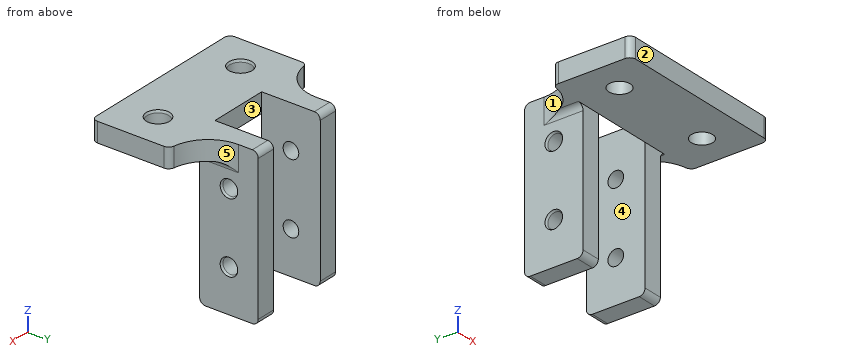
```python
from build123d import *

# Parameters (mm, degrees)
SKETCH1_W                           = 45
SKETCH1_H                           = 20
BOSS_EXTRUDE1_DEPTH                 = 5
BOSS_EXTRUDE2_DEPTH                 = 15
F_4_0_4_DIAMETER_HOLE1_AT_2_COUNT   = 2
F_4_0_4_DIAMETER_HOLE1_AT_2_PITCH   = 18
F_5_5_5_5_DIAMETER_HOLE2_AT_2_COUNT = 2
F_5_5_5_5_DIAMETER_HOLE2_AT_2_PITCH = 27
FILLET1_R                           = 10
FILLET2_R                           = 1.5


with BuildPart() as part:
    # Sketch1 → Boss-Extrude1 (new body)
    with BuildSketch(Plane.XY):
        Rectangle(SKETCH1_W, SKETCH1_H)
    extrude(amount=BOSS_EXTRUDE1_DEPTH)

    # Sketch3 → Boss-Extrude2 (add)
    with BuildSketch(Plane(origin=(0, 10, 0), x_dir=(1, 0, 0), z_dir=(0, 1, 0))):
        Polygon((-7.65, 0), (-7.65, -5), (-12.65, -5), (-12.65, 35), (-7.65, 35), align=None)
        Polygon((7.65, -5), (12.65, -5), (12.65, 35), (7.65, 35), (7.65, 0), align=None)
    extrude(amount=BOSS_EXTRUDE2_DEPTH)

    # Sketch8 → Ø4.0 (4) Diameter Hole1 (revolve, cut)
    with BuildSketch(Plane(origin=(-12.65, 17.5, -24), x_dir=(0, 0, 1), z_dir=(0, 1, 0))):
        Polygon((0, 0), (0, 5), (2, 5), (2, 0.603553391), (2.25, 0), align=None)
    f_4_0_4_diameter_hole1 = revolve(axis=Axis((-19, 17.5, -24), (1, 0, 0)), mode=Mode.SUBTRACT)

    # Ø4.0 (4) Diameter Hole1 at 2: Ø4.0 (4) Diameter Hole1 ×2
    with Locations(*[(0, 0, i * F_4_0_4_DIAMETER_HOLE1_AT_2_PITCH) for i in range(1, F_4_0_4_DIAMETER_HOLE1_AT_2_COUNT)]):
        add(f_4_0_4_diameter_hole1, mode=Mode.SUBTRACT)

    # Mirror3: Ø4.0 (4) Diameter Hole1 across plane
    add(f_4_0_4_diameter_hole1.mirror(Plane(origin=(0, 0, 0), x_dir=(0, 0, 1), z_dir=(1, 0, 0))), mode=Mode.SUBTRACT)

    # Mirror3 copy 1 sketch → Mirror3 copy 1 (revolve, cut)
    with BuildSketch(Plane(origin=(12.65, 17.5, -6), x_dir=(0, 0, 1), z_dir=(0, 1, 0))):
        Polygon((0, 0), (0, -5), (2, -5), (2, -0.603553391), (2.25, 0), align=None)
    revolve(axis=Axis((19, 17.5, -6), (1, 0, 0)), mode=Mode.SUBTRACT)

    # Sketch12 → Ø5.5 (5.5) Diameter Hole2 (revolve, cut)
    with BuildSketch(Plane(origin=(13.5, 0, 5), x_dir=(0, -1, 0), z_dir=(1, 0, 0))):
        Polygon((0, 0), (0, 5), (2.75, 5), (2.75, 0.603553391), (3, 0), align=None)
    f_5_5_5_5_diameter_hole2 = revolve(axis=Axis((13.5, 0, 11.35), (0, 0, -1)), mode=Mode.SUBTRACT)

    # Ø5.5 (5.5) Diameter Hole2 at 2: Ø5.5 (5.5) Diameter Hole2 ×2
    with Locations(*[(-i * F_5_5_5_5_DIAMETER_HOLE2_AT_2_PITCH, 0, 0) for i in range(1, F_5_5_5_5_DIAMETER_HOLE2_AT_2_COUNT)]):
        add(f_5_5_5_5_diameter_hole2, mode=Mode.SUBTRACT)

    # Fillet1
    # the kernel refuses this fillet: 10 mm, written as the material it adds along each edge
    with BuildSketch(Plane(origin=(12.65, 10, 5), x_dir=(1, 0, 0), z_dir=(0, 0, -1))) as fillet1_piece_1:
        with BuildLine():
            CenterArc((10, -9.998874937), FILLET1_R, 90.859468925, 89.140531075)
            Line((0, -9.998874937), (0, 0))
            Line((0, 0), (9.85, 0))
        make_face()
    extrude(amount=5)
    with BuildSketch(Plane(origin=(-12.65, 10, 5), x_dir=(-1, 0, 0), z_dir=(0, 0, -1))) as fillet1_piece_2:
        with BuildLine():
            CenterArc((10, 9.998874937), FILLET1_R, 180, 89.140531075)
            Line((0, 9.998874937), (0, 0))
            Line((0, 0), (9.85, 0))
        make_face()
    extrude(amount=5)

    # Fillet2
    fillet2_edges = [part.edges().sort_by_distance(p)[0] for p in [
        (-10.15, 10, -35),
        (-10.15, 25, -35),
        (-10.15, 25, 5),
        (10.15, 10, -35),
        (10.15, 25, 5),
        (10.15, 25, -35),
        (22.5, -10, 2.5),
        (-22.5, -10, 2.5),
        (-22.5, 10, 2.5),
        (22.5, 10, 2.5),
        (12.65, 14.999437468, 0),
        (-12.65, 14.999437468, 0),
    ]]
    fillet(fillet2_edges, radius=FILLET2_R)


solid = part.part
```
Could you check a few things on this model? Use its own coordinates, in mm. Face numbers are marked on the shaded views. A direction names the side the tool comes from. Round coordinates to 2 decimals unless told otherwise and drop trailing zeros. Loops run counter-clockwise (first coordinate to the right, second up) from the corner with the lowest first, then second, coordinate; pieces in that order, holes last. Notation, with made-up numbers: (12, -26) -> (55, -26) arc R12 cw to (55, -14) -> close; hole circle Ø1 at (76.5, 78). An arc over 180 degrees is marked (long way). One line per question, with ' | ' between items.
(1) For pin 1 Ø1.5 at (y, z) = (13, 0.5) entering from -X; pin 2 Ø2.5 at (y, z) = (17.5, -24) entering from +X; pin 3 Ø7.5 at (y, z) = (19, -18.5) entering from +X; pin 4 Ø3 at (x, z) = (9.5, -11) entering from -Y, each with a flat end and sliding along its axis, tell me the tip position at first contact or that it passes through.
Model answer:
pin 1: stops at x = -16.33 | pin 2: passes through | pin 3: stops at x = 12.65 | pin 4: stops at y = 10
(2) Thinking about a two-plate mould opening in X: for the marked faces 1, 2 and 3, which applies, released by +X, released by -X, zero draft, split by the parting line, or undercut?
Model answer:
face 1: released by -X | face 2: zero draft | face 3: undercut
(3) If we section it at A-A on z = -6: List the corners of the cut face in (x, y) for me.
Model answer:
outline: (-12.65, 10) -> (-7.65, 10) -> (-7.65, 15.5) -> (-12.05, 15.5) -> (-12.65, 15.25) -> close; (-12.65, 19.75) -> (-12.05, 19.5) -> (-7.65, 19.5) -> (-7.65, 25) -> (-12.65, 25) -> close; (7.65, 10) -> (12.65, 10) -> (12.65, 15.25) -> (12.05, 15.5) -> (7.65, 15.5) -> close; (7.65, 19.5) -> (12.05, 19.5) -> (12.65, 19.75) -> (12.65, 25) -> (7.65, 25) -> close
(4) If we section it at D-D on y = 0: List the corners of the cut face in (x, z) for me.
Model answer:
outline: (-22.5, 0) -> (-16.25, 0) -> (-16.25, 4.4) -> (-16.5, 5) -> (-22.5, 5) -> close; (-10.75, 0) -> (10.75, 0) -> (10.75, 4.4) -> (10.5, 5) -> (-10.5, 5) -> (-10.75, 4.4) -> close; (16.25, 0) -> (22.5, 0) -> (22.5, 5) -> (16.5, 5) -> (16.25, 4.4) -> close
(5) If we section it at C-C on z = -14: List the corners of the cut face in (x, y) for me.
Model answer:
outline: (-12.65, 10) -> (-7.65, 10) -> (-7.65, 25) -> (-12.65, 25) -> close; (7.65, 10) -> (12.65, 10) -> (12.65, 25) -> (7.65, 25) -> close
(6) For the marked faces 4 and 5, which set-ups out of +Z, -Z, +X, -X, +Y, -Y let a thin tool reach every point of the face, with its end or its side?
Model answer:
face 4: +Z, -Z, +Y | face 5: +Z, -Z, +X, +Y
(7) If I drill on probe 1 along Z at (x, y) = (10.7, 17.5); probe 2 along X at (y, z) = (0, 2); probe 3 along X at (y, z) = (16.5, -11), over which ranges is the centre line in solid material (lowest first)?
Model answer:
probe 1: z = -35 to -26, -22 to -8, -4 to 5 | probe 2: x = -22.5 to -16.25, -10.75 to 10.75, 16.25 to 22.5 | probe 3: x = -12.65 to -7.65, 7.65 to 12.65
(8) If we section it at B-B on x = 9: List the corners of the cut face in (y, z) for me, and give its area (3 significant figures).
Model answer:
outline: (-10, 0) -> (10, 0) -> (10, -33.5) arc R1.5 ccw to (11.5, -35) -> (23.5, -35) arc R1.5 ccw to (25, -33.5) -> (25, 3.5) arc R1.5 ccw to (23.5, 5) -> (-10, 5) -> close; hole circle Ø4 at (17.5, -24); hole circle Ø4 at (17.5, -6) | area: 673 mm^2
